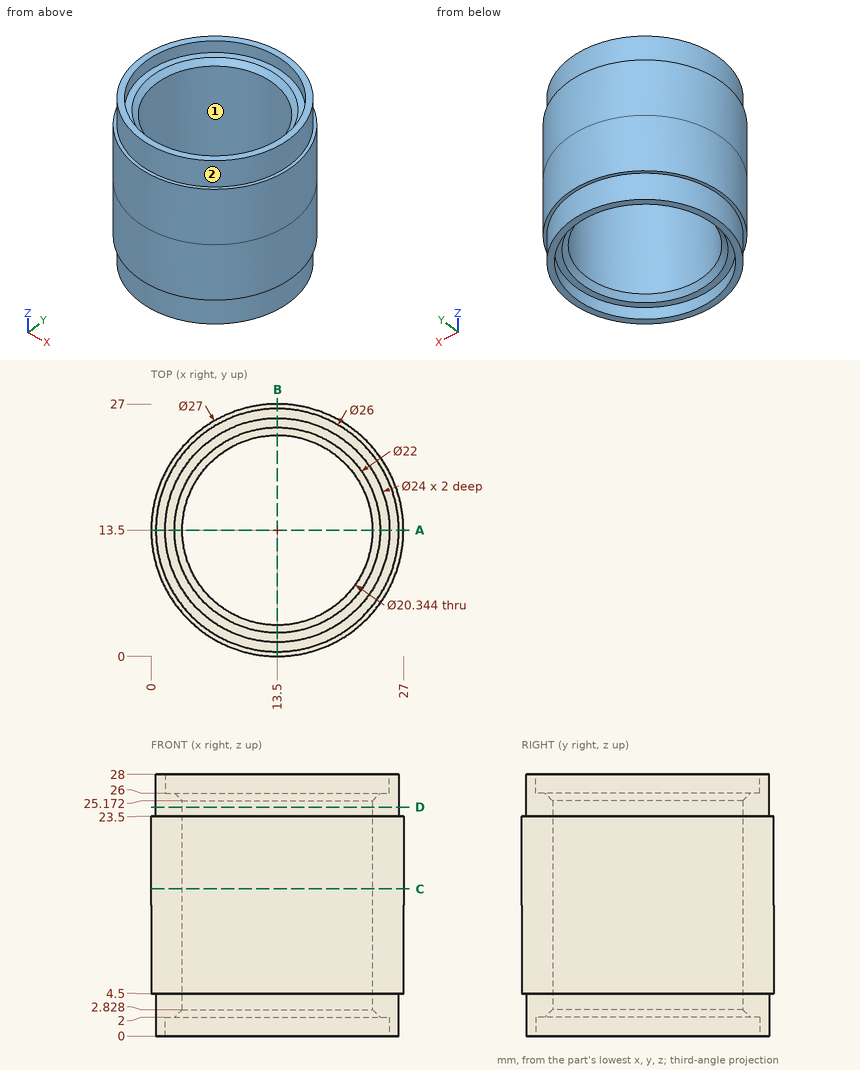
The drawing under review shows one solid part. Ordinate dimensions are in mm from its lowest x, y, z. Coordinates: 2 decimals unless noted, no trailing zeros. Write each loop counter-clockwise with the first axis right and the second up, starting at its lowest first coordinate (ties: lowest second). Pieces come first, ordered by that corner, then holes. Notation, with made-up numbers: (20.5, 6) - (68.5, 6) arc R19 ccw to (68.5, 31) - close; hole circle Ø3 at (-23, 63). An arc over 180 degrees is marked (long way). Put each result on its own line as item: value.
1. Add section A-A, the plane y = 13.5. Give the boundary of the cut face in (x, z).
Values found:
outline: (0, 4.5) - (0.5, 4.5) - (0.5, 0) - (1.5, 0) - (1.5, 2) - (2.5, 2) - (3.33, 2.83) - (3.33, 25.17) - (2.5, 26) - (1.5, 26) - (1.5, 28) - (0.5, 28) - (0.5, 23.5) - (0, 23.5) - close; (23.67, 2.83) - (24.5, 2) - (25.5, 2) - (25.5, 0) - (26.5, 0) - (26.5, 4.5) - (27, 4.5) - (27, 23.5) - (26.5, 23.5) - (26.5, 28) - (25.5, 28) - (25.5, 26) - (24.5, 26) - (23.67, 25.17) - close
2. Mouldability with a two-part tool opening along Y and no side actions: class the marked faces 1 and 2 as released by +Y, released by -Y, zero draft, split by the parting line, or undercut.
Values found:
face 1: undercut
face 2: split by the parting line
3. For pin 1 (7 mm diameter, centred on x = 14.5, y = 8, fed in from +Z); pin 2 (10 mm diameter, centred on y = 6.5, z = 5.5, fed in from +X); pin 3 (6 mm diameter, centred on y = 22, z = 4, fed in from -X); pin 4 (1.5 mm diameter, centred on x = 9.5, y = 23.5, fed in from -Z), all flat-tipped, find the tip position at first contact; note any pin that passes through.
Values found:
pin 1: through
pin 2: x = 26.85
pin 3: x = 1.19
pin 4: z = 2
4. Wall thickness on probe 1 along Y at (x, z) = (13.5, 27.5); probe 2 along Y at (x, z) = (13.5, 16.5); probe 3 along Z at (x, y) = (2.5, 13): over which ranges is each line inside the solid? List them lowest first.
Values found:
probe 1: 0.5 to 1.5, 25.5 to 26.5
probe 2: 0 to 3.33, 23.67 to 27
probe 3: 2 to 26
5. Add section C-C, the plane z = 15.75. Give the boundary of the cut face in (x, y).
Values found:
outline: circle Ø27 at (13.5, 13.5); hole circle Ø20.34 at (13.5, 13.5)
6. Add section D-D, the plane z = 24.5. Give the boundary of the cut face in (x, y), then the cut area to 3 significant figures.
Values found:
outline: circle Ø26 at (13.5, 13.5); hole circle Ø20.34 at (13.5, 13.5)
area: 206 mm²
